Work out the finished part from the listing and answer in its coordinate system (mm). Face numbers are marked on the shaded views. Coordinates: 2 decimals unless noted, no trailing zeros. Write each loop counter-clockwise with the first axis right and the second up, starting at its lowest first coordinate (ties: lowest second). Pieces come first, ordered by that corner, then holes. Notation, with made-up numbers: (-16.5, 56) - (8.5, 56) arc R19 cw to (8.5, 74) - close; hole circle Ø5 at (-30.5, -30.5). An arc over 180 degrees is marked (long way). Use one line per item in the form item = value. Start each with the question number.
Item 1: A cutting plane is placed at D-D (z = 2.5). Write down the section's boundary in (x, y), then the cut area to 3 significant figures.
Item 2: Determine the mould class of the marked faces 1, 2, 3 and 4 for opening direction Y: released by +Y, released by -Y, zero draft, split by the parting line, or undercut.
Item 3: A cutting plane is placed at C-C (x = 4). Write down the section's boundary in (y, z), then the cut area to 3 significant figures.
Item 4: Consider probe 1 along Y at (x, z) = (-14, 2.1); probe 2 along X at (y, z) = (14.5, 1.35); probe 3 along Y at (x, z) = (2.5, 1.65). Determine where each line is inside the solid, lowest interval first.
Item 5: A cutting plane is placed at A-A (x = -14). Write down the section's boundary in (y, z).
Item 6: A cutting plane is placed at B-B (y = 14). Write down the section's boundary in (x, z).
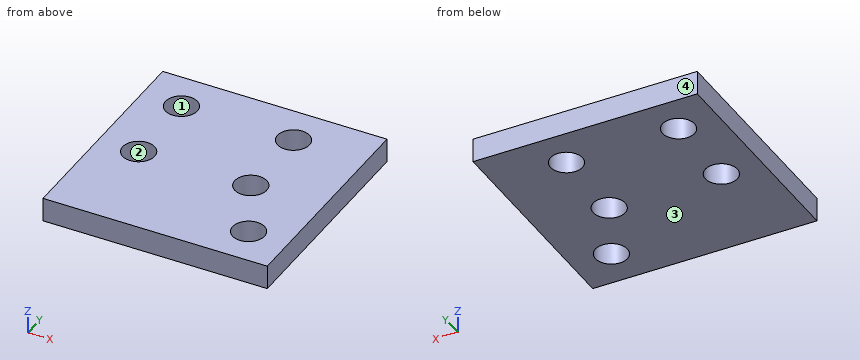
from build123d import *

# Parameters (mm, degrees)
F0_W     = 38
F0_H     = 38
F1_DEPTH = 3
F3_D     = 4
F5_DEPTH = 25


with BuildPart() as f1:
    # F0 (on Top) → F1 (new body)
    with BuildSketch(Plane.XY):
        Rectangle(F0_W, F0_H)
    extrude(amount=F1_DEPTH)

    # F3 (through all)
    with Locations(Plane.XY.offset(3)):
        with Locations((0, 4), (0, 14), (-14, 14), (4, -4), (-14, 4)):
            Hole(F3_D / 2)

    # F4 (on face) → F5 (cut)
    with BuildSketch(Plane.XY.offset(3)):
        Polygon((19, 19), (9, 19), (9, -9), (-19, -9), (-19, -19), (19, -19), align=None)
    extrude(amount=-F5_DEPTH, mode=Mode.SUBTRACT)


solid = f1.part
Answer:
q1.outline = (-19, -9) - (9, -9) - (9, 19) - (-19, 19) - close; hole circle Ø4 at (-14, 4); hole circle Ø4 at (-14, 14); hole circle Ø4 at (0, 4); hole circle Ø4 at (0, 14); hole circle Ø4 at (4, -4)
q1.area = 721 mm²
q2.face_1 = undercut
q2.face_2 = undercut
q2.face_3 = zero draft
q2.face_4 = released by +Y
q3.outline = (-9, 0) - (-6, 0) - (-6, 3) - (-9, 3) - close; (-2, 0) - (19, 0) - (19, 3) - (-2, 3) - close
q3.area = 72.0 mm²
q4.probe_1 = -9 to 2, 6 to 12, 16 to 19
q4.probe_2 = -19 to -15.94, -12.06 to -1.94, 1.94 to 9
q4.probe_3 = -9 to -5.32, -2.68 to 19
q5.outline = (-9, 0) - (2, 0) - (2, 3) - (-9, 3) - close; (6, 0) - (12, 0) - (12, 3) - (6, 3) - close; (16, 0) - (19, 0) - (19, 3) - (16, 3) - close
q6.outline = (-19, 0) - (-16, 0) - (-16, 3) - (-19, 3) - close; (-12, 0) - (-2, 0) - (-2, 3) - (-12, 3) - close; (2, 0) - (9, 0) - (9, 3) - (2, 3) - close
